Design review of the part built by this model. Coordinates are the model's own, in mm. Coordinates: 2 decimals unless noted, no trailing zeros. Write each loop counter-clockwise with the first axis right and the second up, starting at its lowest first coordinate (ties: lowest second). Pieces come first, ordered by that corner, then holes. Notation, with made-up numbers: M 55.5,1.5 L 91.5,1.5 A28 cw 91.5,22.5 Z; hole C 61.5,-5 d1. An arc over 180 degrees is marked long. Write item = value, one per line.
Autodesk Inventor part; units mm, degrees
ref_plane "YZ Plane" through (0, 0, 0) normal (1, 0, 0) x (0, 1, 0)
ref_plane "XZ Plane" through (0, 0, 0) normal (0, 1, 0) x (-1, 0, 0)
ref_plane "XY Plane" through (0, 0, 0) normal (0, 0, 1) x (1, 0, 0)
sketch "Sketch1" plane through (0, 0, 0) normal (0, 1, 0) x (-1, 0, 0)
  line L0 (0, 0) -> (-100, 0)
  line L1 (-100, 0) -> (-100, -150)
  line L2 (-100, -150) -> (0, -150)
  line L3 (0, -150) -> (0, 0)
  dimension "d0" = 150
  dimension "d1" = 100
extrude "Extrusion1" add sketch "Sketch1" along normal blind 5
sketch "Sketch2" plane through (0, 5, 0) normal (0, 1, 0) x (1, 0, 0)
  circle A0 centre (65.8462, 111.6036) radius 1.5
  circle A1 centre (61.6036, 115.8462) radius 1.5
  circle A2 centre (38.3964, 115.8462) radius 1.5
  circle A3 centre (34.1538, 111.6036) radius 1.5
  circle A4 centre (34.1538, 88.3964) radius 1.5
  circle A5 centre (38.3964, 84.1538) radius 1.5
  circle A6 centre (61.6036, 84.1538) radius 1.5
  circle A7 centre (65.8462, 88.3964) radius 1.5
  point P0 (0, 0)
extrude "Extrusion2" cut sketch "Sketch2" against normal blind 5
sketch "Sketch3" plane through (0, 5, 0) normal (0, 1, 0) x (1, 0, 0)
  circle A0 centre (5, 145) radius 1.5
  circle A1 centre (5, 5) radius 1.5
  circle A2 centre (95, 5) radius 1.5
  point P0 (0, 0)
extrude "Extrusion3" cut sketch "Sketch3" against normal blind 5
equation "\"d2\" = woodThickness"
equation "\"d4\" = woodThickness"
equation "\"d6\" = woodThickness"
equation "\"bladeLenghtFlexRatio\" = 0.05"
equation "\"bladeThickness\" = 1"
equation "\"woodThickness\" = 5"
equation "\"colRadius\" = 3"
equation "\"M3Hole\" = 3"
properties part number "FlexBlockWheelSupport"
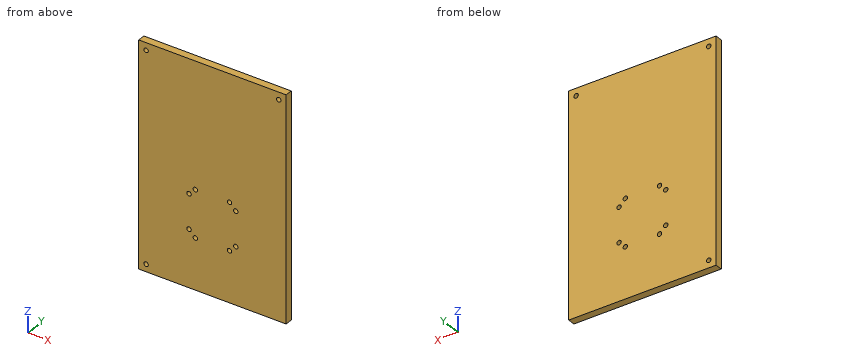
Q1. Consider section B-B, the plane z = -5. State the section outline as (x, y) points, and give its area (3 significant figures).
Check result:
outline = M 0,0 L 3.5,0 L 3.5,5 L 0,5 Z; M 6.5,0 L 93.5,0 L 93.5,5 L 6.5,5 Z; M 96.5,0 L 100,0 L 100,5 L 96.5,5 Z
area = 470 mm²
Q2. Consider section D-D, the plane x = 95. State the section outline as (y, z) points.
Check result:
outline = M 0,-150 L 5,-150 L 5,-6.5 L 0,-6.5 Z; M 0,-3.5 L 5,-3.5 L 5,0 L 0,0 Z
Q3. Consider section C-C, the plane z = -145. State the section outline as (x, y) points, and give its area (3 significant figures).
Check result:
outline = M 0,0 L 3.5,0 L 3.5,5 L 0,5 Z; M 6.5,0 L 100,0 L 100,5 L 6.5,5 Z
area = 485 mm²
Q4. Wall thickness on line 1 (Z direction, x = 5, y = 1.8); line 2 (Z direction, x = 61, y = 2.5); line 3 (X direction, y = 1.05, z = -116.5): over which ranges is each line inside the solid? List them lowest first.
Check result:
line_1 = -150 to -146.5, -143.5 to -6.5, -3.5 to 0
line_2 = -150 to -117.22, -114.47 to -85.53, -82.78 to 0
line_3 = 0 to 37.05, 39.75 to 60.25, 62.95 to 100
Q5. For P1, Ø4, axis at x = 95, z = -5, coming from the +Y side; P2, Ø1.8, axis at x = 61.6, z = -115.85, coming from the -Y side, all flat-tipped, find the tip position at first contact; note any pin that passes through.
Check result:
P1 = 5
P2 = through
Q6. Consider section A-A, the plane x = 5. State the section outline as (y, z) points.
Check result:
outline = M 0,-150 L 5,-150 L 5,-146.5 L 0,-146.5 Z; M 0,-143.5 L 5,-143.5 L 5,-6.5 L 0,-6.5 Z; M 0,-3.5 L 5,-3.5 L 5,0 L 0,0 Z
